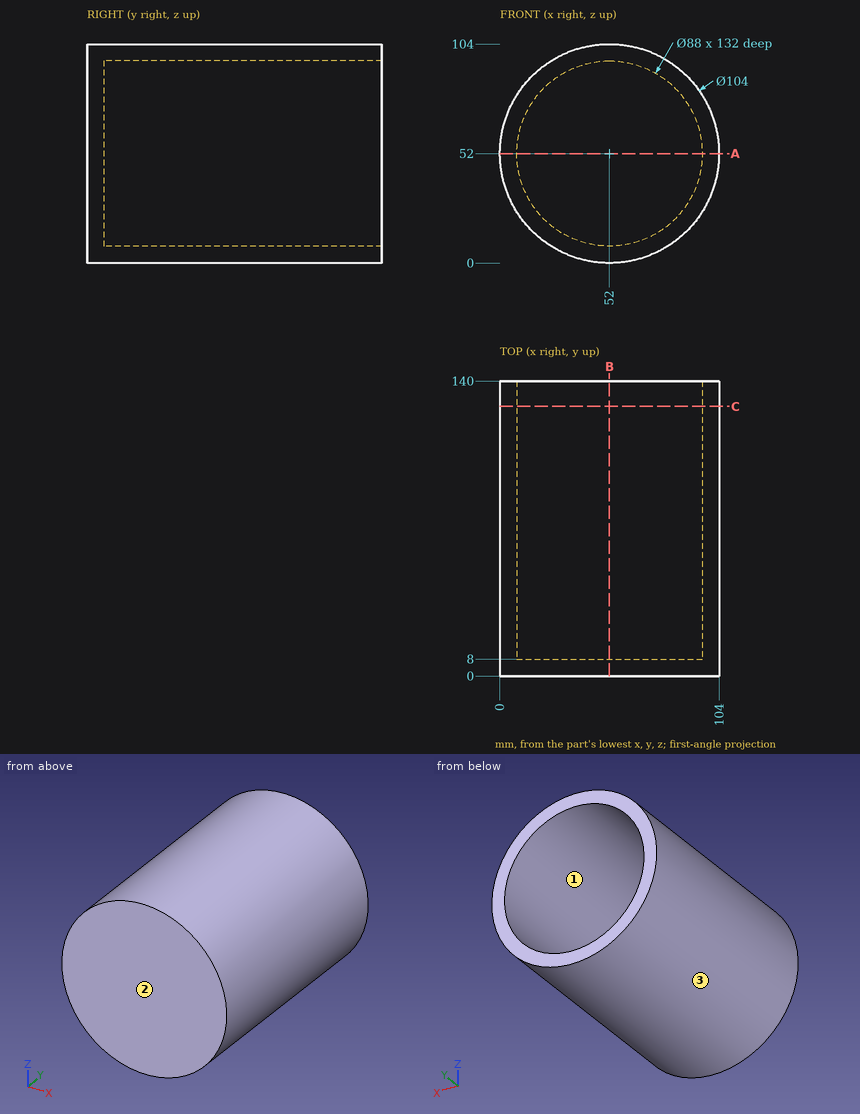
Verification items for this drawing (mm, ordinates from the low corner). Coordinates: 2 decimals unless noted, no trailing zeros. Write each loop counter-clockwise with the first axis right and the second up, starting at its lowest first coordinate (ties: lowest second). Pieces come first, ordered by that corner, then holes. Notation, with made-up numbers: (19.25, 16) -> (69.25, 16) arc R21 ccw to (69.25, 33) -> close; hole circle Ø9 at (50.5, 47). An arc over 180 degrees is marked (long way). One line per item, written item: value. Start each with the question number.
Q1. Thickness scan on L1, parallel to X at y = 86, z = 52; L2, parallel to Y at x = 67, z = 21. Record the ranges inside material, lowest first. Write a range as from..to.
Q2. Mould release check, pull along Z, two halves, no side actions. Record for the marked faces 1, 2 and 3: pulls with the +Z half, pulls with the -Z half, needs draft (parallel to the pull), parting line crosses it, or undercut.
Q3. Cross-section at C-C on y = 128. Enter the section's corners in (x, z).
Q4. Cross-section at B-B on x = 52. Enter the section's corners in (y, z).
Q5. Cross-section at A-A on z = 52. Enter the section's corners in (x, y).
Q6. Go/stop test with flat-tipped pins: P1, Ø5, axis at x = 36, z = 87.5, coming from the +Y side; P2, Ø12, axis at y = 16.5, z = 25.5, coming from the +X side; P3, Ø1.5, axis at y = 94.5, z = 64.5, coming from the +X side. Record where each tip stops, or that it passes through.
Checked values:
1. L1: x = 0..8, 96..104
1. L2: y = 0..8
2. face 1: undercut
2. face 2: needs draft
2. face 3: parting line crosses it
3. outline: circle Ø104 at (52, 52); hole circle Ø88 at (52, 52)
4. outline: (0, 0) -> (140, 0) -> (140, 8) -> (8, 8) -> (8, 96) -> (140, 96) -> (140, 104) -> (0, 104) -> close
5. outline: (0, 0) -> (104, 0) -> (104, 140) -> (96, 140) -> (96, 8) -> (8, 8) -> (8, 140) -> (0, 140) -> close
6. P1: stops at y = 8
6. P2: stops at x = 99.79
6. P3: stops at x = 102.66
